The model under review builds one solid part; all positions refer to its coordinate system, in mm. Coordinates: 2 decimals unless noted, no trailing zeros. Write each loop counter-clockwise with the first axis right and the second up, starting at its lowest first coordinate (ties: lowest second). Pieces come first, ordered by that corner, then holes. Notation, with made-up numbers: (28, -34.5) - (87, -34.5) arc R18 cw to (87, -4.5) - close; hole circle Ø10 at (-17, 28). An arc over 180 degrees is marked (long way). Return JSON: item names as keys, results as strings. Group by question number.
(1) To check wall thickness, follow L1, parallel to Y at x = -34, z = -1.65; L2, parallel to Y at x = 34, z = -3.2; L3, parallel to X at y = 21, z = -1.7. State the ranges of each line that lie inside material, in increasing order. Write a range as from..to.
(2) We need section A-A on x = 0. State the section outline as (y, z) points.
(3) For pin 1 Ø1.2 at (y, z) = (44.5, -2) entering from +X; pin 2 Ø1 at (y, z) = (-4, -1) entering from +X; pin 3 Ø1.2 at (y, z) = (33, -2) entering from -X, all flat-tipped, find the tip position at first contact; note any pin that passes through.
(4) We need section C-C on z = -2.4. State the section outline as (x, y) points, then the cut area to 3 significant figures.
(5) We need section D-D on x = 34. State the section outline as (y, z) points.
(6) We need section B-B on y = 0. State the section outline as (x, z) points.
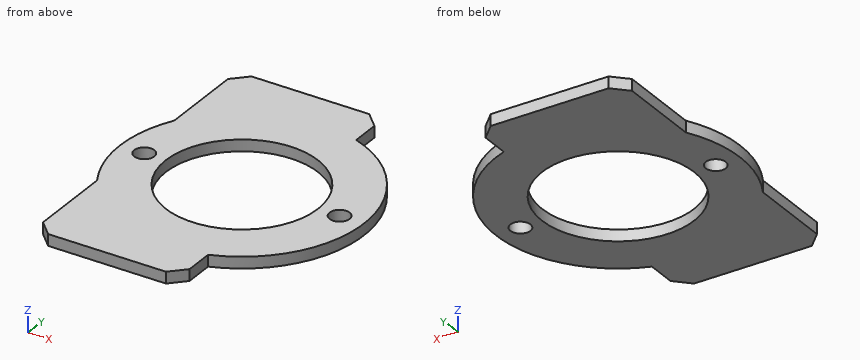
```python
from build123d import *

# Parameters (mm, degrees)
SKETCH1_R           = 42.5
SKETCH1_R_2         = 26.5
SKETCH1_R_3         = 3.5
BOSS_EXTRUDE1_DEPTH = 4
BOSS_EXTRUDE2_DEPTH = 4
CHAMFER1_SIZE       = 5


with BuildPart() as part:
    # Sketch1 → Boss-Extrude1 (new body)
    with BuildSketch(Plane.XY):
        Circle(SKETCH1_R)
        Circle(SKETCH1_R_2, mode=Mode.SUBTRACT)
        with Locations((34, 0)):
            Circle(SKETCH1_R_3, mode=Mode.SUBTRACT)
        with Locations((-34, 0)):
            Circle(SKETCH1_R_3, mode=Mode.SUBTRACT)
    extrude(amount=-BOSS_EXTRUDE1_DEPTH)

    # Sketch2 → Boss-Extrude2 (add)
    with BuildSketch(Plane.XY):
        Polygon((-37, 55), (-37, 20.910523666), (14, 40.127920454), (14, 55), align=None)
        Polygon((-37, -55.188269352), (-37, -20.910523666), (14, -40.127920454), (14, -55.188269352), align=None)
    extrude(amount=-BOSS_EXTRUDE2_DEPTH)

    # Chamfer1
    chamfer1_edges = [part.edges().sort_by_distance(p)[0] for p in [
        (-37, 55, -2),
        (14, 55, -2),
        (14, -55.188269352, -2),
        (-37, -55.188269352, -2),
    ]]
    chamfer(chamfer1_edges, length=CHAMFER1_SIZE)


solid = part.part
```
Ans:
{
 "1": {"L1": "-53.19..-3.5, 3.5..53", "L2": "-25.5..-3.5, 3.5..25.5", "L3": "-37..-16.16, 16.16..36.95"},
 "2": {"outline": "(-55.19, -4) - (-26.5, -4) - (-26.5, 0) - (-55.19, 0) - close; (26.5, -4) - (55, -4) - (55, 0) - (26.5, 0) - close"},
 "3": {"pin 1": "x = 14", "pin 2": "x = 42.36", "pin 3": "x = -37"},
 "4": {"outline": "(-37, -50.19) - (-32, -55.19) - (9, -55.19) - (14, -50.19) - (14, -40.13) arc R42.5 ccw to (14, 40.13) - (14, 50) - (9, 55) - (-32, 55) - (-37, 50) - (-37, 20.91) arc R42.5 ccw to (-37, -20.91) - close; hole circle Ø7 at (-34, 0); hole circle Ø53 at (0, 0); hole circle Ø7 at (34, 0)", "area": "5,110 mm²"},
 "5": {"outline": "(-25.5, -4) - (-3.5, -4) - (-3.5, 0) - (-25.5, 0) - close; (3.5, -4) - (25.5, -4) - (25.5, 0) - (3.5, 0) - close"},
 "6": {"outline": "(-42.5, -4) - (-37.5, -4) - (-37.5, 0) - (-42.5, 0) - close; (-30.5, -4) - (-26.5, -4) - (-26.5, 0) - (-30.5, 0) - close; (26.5, -4) - (30.5, -4) - (30.5, 0) - (26.5, 0) - close; (37.5, -4) - (42.5, -4) - (42.5, 0) - (37.5, 0) - close"}
}
